Geometry: final body of the model. Coordinates: model frame, mm. Face numbers are marked on the shaded views. A direction names the side the tool comes from. Coordinates: 2 decimals unless noted, no trailing zeros. Order: outer loops, then holes, each group sorted by start corner. A loop starts at its lowest first (then second) coordinate and runs counter-clockwise, first axis right, second up. Notation, with made-up numbers: (35.5, 32) -> (56.5, 32) arc R19 cw to (56.5, 53) -> close; hole circle Ø10 at (43.25, -11.75). An arc over 180 degrees is marked (long way). Use one line per item in the form item = value.
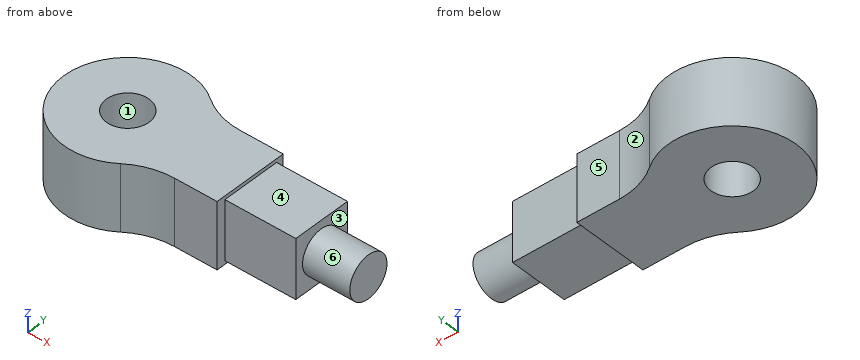
```python
from build123d import *

# Parameters (mm, degrees)
SKETCH5_R           = 9
BOSS_EXTRUDE7_DEPTH = 28
SKETCH6_OUTSIDE_W   = 58.478
SKETCH6_OUTSIDE_H   = 84.478
SKETCH6_OUTSIDE_R   = 9
CUT_EXTRUDE1_DEPTH  = 20
SKETCH7_OUTSIDE_W   = 58.478
SKETCH7_OUTSIDE_H   = 84.478
SKETCH7_OUTSIDE_W_2 = 25
SKETCH7_OUTSIDE_H_2 = 25
CUT_EXTRUDE3_DEPTH  = 30


with BuildPart() as part:
    # Sketch5 → Boss-Extrude7 (new body)
    with BuildSketch(Plane.XY):
        with BuildLine():
            Line((33.660065359, 16), (101.748563171, 16))
            Line((101.748563171, 16), (101.748563171, -16))
            Line((101.748563171, -16), (33.660065359, -16))
            ThreePointArc((33.660065359, -16), (24.341154196, -17.484076471), (15.944241486, -21.789473684))
            ThreePointArc((15.944241486, -21.789473684), (-27, 0), (15.944241486, 21.789473684))
            ThreePointArc((15.944241486, 21.789473684), (24.341154196, 17.484076471), (33.660065359, 16))
        make_face()
        Circle(SKETCH5_R, mode=Mode.SUBTRACT)
    extrude(amount=BOSS_EXTRUDE7_DEPTH)

    # Sketch6 outside → Cut-Extrude1 (cut)
    with BuildSketch(Plane(origin=(101.748563171, 0, 0), x_dir=(0, 0, -1), z_dir=(1, 0, 0))):
        with Locations((-14, 0)):
            Rectangle(SKETCH6_OUTSIDE_W, SKETCH6_OUTSIDE_H)
        with Locations((-14, 0)):
            Circle(SKETCH6_OUTSIDE_R, mode=Mode.SUBTRACT)
    extrude(amount=-CUT_EXTRUDE1_DEPTH, mode=Mode.SUBTRACT)

    # Sketch7 outside → Cut-Extrude3 (cut)
    with BuildSketch(Plane(origin=(81.748563171, 0, 0), x_dir=(0, 0, -1), z_dir=(1, 0, 0))):
        with Locations((-14, 0)):
            Rectangle(SKETCH7_OUTSIDE_W, SKETCH7_OUTSIDE_H)
        with Locations((-14, 0.259981409)):
            Rectangle(SKETCH7_OUTSIDE_W_2, SKETCH7_OUTSIDE_H_2, mode=Mode.SUBTRACT)
    extrude(amount=-CUT_EXTRUDE3_DEPTH, mode=Mode.SUBTRACT)


solid = part.part
```
1) Pull-direction query (Y, two-part tool) for the marked faces 1, 2 and 3; classes: released by +Y, released by -Y, zero draft, split by the parting line, or undercut.
Results found:
face_1 = undercut
face_2 = released by +Y
face_3 = zero draft
2) Contact query for flat-ended pins moving along their axis: P1, Ø3, axis at y = 4.5, z = 5.5, coming from the -X side; P2, Ø12.5, axis at x = 60.5, z = 14, coming from the -Y side; P3, Ø3, axis at x = 75, y = -9, coming from the -Z side. Output: stop coordinate, or through.
Results found:
P1 = -26.83
P2 = -12.24
P3 = 1.5
3) Section B-B, the plane z = 24.5. Output: boundary loops of the cut face in (x, y).
Results found:
outline = (15.94, -21.79) arc R30 cw to (33.66, -16) -> (51.75, -16) -> (51.75, -12.24) -> (81.75, -12.24) -> (81.75, 12.76) -> (51.75, 12.76) -> (51.75, 16) -> (33.66, 16) arc R30 cw to (15.94, 21.79) arc R27 ccw (long way) to start; hole circle Ø18 at (0, 0)
4) Section A-A, the plane y = 0. Output: boundary loops of the cut face in (x, z).
Results found:
outline = (-27, 0) -> (-9, 0) -> (-9, 28) -> (-27, 28) -> close; (9, 0) -> (51.75, 0) -> (51.75, 1.5) -> (81.75, 1.5) -> (81.75, 5) -> (101.75, 5) -> (101.75, 23) -> (81.75, 23) -> (81.75, 26.5) -> (51.75, 26.5) -> (51.75, 28) -> (9, 28) -> close
5) Section C-C, the plane x = 0. Output: boundary loops of the cut face in (y, z).
Results found:
outline = (-27, 0) -> (-9, 0) -> (-9, 28) -> (-27, 28) -> close; (9, 0) -> (27, 0) -> (27, 28) -> (9, 28) -> close
6) Material intervals for probe 1 along Y at (x, z) = (0, 10.75); probe 2 along Y at (x, z) = (80.5, 15.5); probe 3 along Z at (x, y) = (59.5, -11), sorted ascending. Write a range as from..to.
Results found:
probe_1 = -27..-9, 9..27
probe_2 = -12.24..12.76
probe_3 = 1.5..26.5
7) Access query for the marked faces 4, 5 and 6. Directions: +Z, -Z, +X, -X, +Y, -Y. A direction counts if a zero-diameter tool reaches every point of the face in a straight line with its end or side. Return the directions, or none.
Results found:
face_4 = +Z, +X, +Y, -Y
face_5 = +Z, -Z, +X, +Y
face_6 = +X
8) Section D-D, the plane x = 45. Output: boundary loops of the cut face in (y, z), and give its area (3 significant figures).
Results found:
outline = (-16, 0) -> (16, 0) -> (16, 28) -> (-16, 28) -> close
area = 896 mm2
